```python
from build123d import *

# Parameters (mm, degrees)
F0_W          = 150
F0_H          = 150
F1_DEPTH      = 80
F3_W          = 10
F3_H          = 130
F4_DEPTH      = 62.5
F4_DEPTH_BACK = 62.5
F5_R          = 7.25
F6_DEPTH      = 7


with BuildPart() as f1:
    # F0 (on Right) → F1 (new body)
    with BuildSketch(Plane.YZ):
        with Locations((75, 75)):
            Rectangle(F0_W, F0_H)
    extrude(amount=F1_DEPTH)

    # F3 (on mid) → F4 (cut, two sides)
    with BuildSketch(Plane.XZ.offset(-75)) as f4_sk:
        with Locations((75, 75)):
            Rectangle(F3_W, F3_H)
        with BuildLine():
            Line((70, 10), (70, 140))
            ThreePointArc((70, 140), (5, 75), (70, 10))
        make_face()
    extrude(amount=-F4_DEPTH, mode=Mode.SUBTRACT)
    extrude(f4_sk.sketch, amount=F4_DEPTH_BACK, mode=Mode.SUBTRACT)

    # F5 (on face) → F6 (cut)
    with BuildSketch(Plane.XZ.offset(-137.5)):
        with Locations((62.25, 75)):
            Circle(F5_R)
    extrude(amount=-F6_DEPTH, mode=Mode.SUBTRACT)

    # F7: F1 across plane


with BuildPart() as f1_1:
    add(f1.part)
    add(f1.part.mirror(Plane(origin=(40, 75, 75), x_dir=(1, 0, 0), z_dir=(0, -1, 0))), mode=Mode.INTERSECT)


solid = f1_1.part
```
Design review of the part built by this model. Coordinates are the model's own, in mm. A direction names the side the tool comes from. Give positions to 0.01 mm unless a question says otherwise; leave off trailing zeros. Write each loop counter-clockwise with the first axis right and the second up, starting at its lowest first coordinate (ties: lowest second). Pieces come first, ordered by that corner, then holes.
(1) Add section B-B (y = 53). Give the boundary of the cut face in (x, z).
Checked values:
outline: (0, 0) - (80, 0) - (80, 10) - (70, 10) arc R65 cw to (70, 140) - (80, 140) - (80, 150) - (0, 150) - close
(2) Tool access review of faces 1 (the face through (75, 74, 10)), 2 (the face through (60.68, 9.05, 67.92)), 3 (the face through (39, 0, 74)): name each direction out of +Z, -Z, +X, -X, +Y, -Y from which nothing blocks a thin tool from reaching the whole face with its end or side.
Checked values:
face 1: +X
face 2: none
face 3: +Z, -Z, +X, -X, -Y
(3) Wall thickness on line 1 along Y through (x, z) = (16, 68.5); line 2 along Z through (x, y) = (62.25, 9.5); line 3 along Z through (x, y) = (53, 95.5): over which ranges is each line inside the solid? List them lowest first.
Checked values:
line 1: y = 0 to 12.5, 137.5 to 150
line 2: z = 0 to 67.75, 82.25 to 150
line 3: z = 0 to 12.26, 137.74 to 150
(4) Add section D-D (x = 67.5). Give the boundary of the cut face in (y, z), and give its area (3 significant figures).
Checked values:
outline: (0, 0) - (150, 0) - (150, 150) - (0, 150) - close; hole (5.5, 70) - (12.5, 70) - (12.5, 10.05) - (137.5, 10.05) - (137.5, 70) - (144.5, 70) - (144.5, 80) - (137.5, 80) - (137.5, 139.95) - (12.5, 139.95) - (12.5, 80) - (5.5, 80) - close
area: 6,120 mm2
(5) Clearance check with a flat-ended pin moving along its axis: pin 1 Ø3 at (y, z) = (43.5, 35.5) entering from +X. State where the tip first meets the part, or that it passes through.
Checked values:
pin 1: stops at x = 19.56
(6) Add section C-C (z = 75). Give the boundary of the cut face in (x, y), and give its area (3 significant figures).
Checked values:
outline: (0, 0) - (80, 0) - (80, 12.5) - (69.5, 12.5) - (69.5, 5.5) - (55, 5.5) - (55, 12.5) - (5, 12.5) - (5, 137.5) - (55, 137.5) - (55, 144.5) - (69.5, 144.5) - (69.5, 137.5) - (80, 137.5) - (80, 150) - (0, 150) - close
area: 2,420 mm2
(7) Mouldability with a two-part tool opening along Z and no side actions: class faces 4 (the face through (80, 141, 76)), 5 (the face through (39, 74, 150)), 6 (the face through (62, 5.5, 75)), 7 (the face through (39, 74, 0)) as +Z half, -Z half, draft (parallel to the pull), parting line (faces both ways), or undercut.
Checked values:
face 4: draft
face 5: +Z half
face 6: undercut
face 7: -Z half
(8) Add section A-A (x = 10). Give the boundary of the cut face in (y, z), and give its area (4 significant figures).
Checked values:
outline: (0, 0) - (150, 0) - (150, 150) - (0, 150) - close; hole (12.5, 50) - (137.5, 50) - (137.5, 100) - (12.5, 100) - close
area: 16,250 mm2
